```python
from build123d import *

# Parameters (mm, degrees)
F1_DEPTH        = 127
F3_DEPTH        = 25.4
F5_DEPTH        = 25.4
F12_DEPTH       = 3.1760001
F14_D           = 7.112
F14_CBORE_D     = 19.05
F14_CBORE_DEPTH = 6.35
F15_R           = 7.112
F15_R_2         = 4.445
F16_DEPTH       = 3.175
F17_R           = 7.112
F17_R_2         = 4.445
F18_DEPTH       = 3.175


with BuildPart() as f1:
    # F0 (on Top) → F1 (new body)
    with BuildSketch(Plane.XY):
        Polygon((-10.5701125115, 27.1786895925), (-17.3647849097, 0), (-14.0920698193, 0), (-8.0911474212, 24.0036895925), (8.0911474212, 24.0036895925), (14.0920698193, 0), (17.3647849097, 0), (10.5701125115, 27.1786895925), align=None)
    extrude(amount=F1_DEPTH)

    # F2 (on face) → F3 (join)
    with BuildSketch(Plane(origin=(0, 0, 0), x_dir=(1, 0, 0), z_dir=(0, 0, -1))):
        Polygon((8.0911474212, -24.0036895925), (14.0920698193, 0), (-14.0920698193, 0), (-8.0911474212, -24.0036895925), align=None)
        Polygon((17.3647849097, 0), (14.0920698193, 0), (8.0911474212, -24.0036895925), (-8.0911474212, -24.0036895925), (-14.0920698193, 0), (-17.3647849097, 0), (-10.5701125115, -27.1786895925), (10.5701125115, -27.1786895925), align=None)
    extrude(amount=F3_DEPTH)

    # F4 (on face) → F5 (join)
    with BuildSketch(Plane.XY.offset(127)):
        Polygon((-8.0911474212, 24.0036895925), (-14.0920698193, 0), (14.0920698193, 0), (8.0911474212, 24.0036895925), align=None)
        Polygon((-17.3647849097, 0), (-14.0920698193, 0), (-8.0911474212, 24.0036895925), (8.0911474212, 24.0036895925), (14.0920698193, 0), (17.3647849097, 0), (10.5701125115, 27.1786895925), (-10.5701125115, 27.1786895925), align=None)
    extrude(amount=F5_DEPTH)

    # F6 (on face) → F8 section 0
    with BuildSketch(Plane(origin=(16.3433269738, 4.0858317435, 0), x_dir=(-0.242535625, 0.9701425001, 0), z_dir=(0.9701425001, 0.242535625, 0))):
        Polygon((-4.2115789617, 158.75), (-4.2115789617, 152.4), (23.8035730273, 152.4), align=None)
    # F7 (on face) → F8 section 1
    with BuildSketch(Plane(origin=(-16.3433269738, 4.0858317435, 0), x_dir=(-0.242535625, -0.9701425001, 0), z_dir=(-0.9701425001, 0.242535625, 0))):
        Polygon((-23.8035730273, 152.4), (4.2115789617, 152.4), (4.2115789617, 158.75), align=None)
    loft()

    # F10 (on face) → F11 section 0
    with BuildSketch(Plane(origin=(-13.2631245358, 3.315781134, 0), x_dir=(0.242535625, 0.9701425001, 0), z_dir=(0.9701425001, -0.242535625, 0))):
        Polygon((-3.4178289617, 6.35), (-3.4178289617, 0), (21.324607937, 0), align=None)
    # F9 (on face) → F11 section 1
    with BuildSketch(Plane(origin=(13.2631245358, 3.315781134, 0), x_dir=(0.242535625, -0.9701425001, 0), z_dir=(-0.9701425001, -0.242535625, 0))):
        Polygon((-21.324607937, 0), (3.4178289617, 0), (3.4178289617, 6.35), align=None)
    loft()

    # F12 (cut, through all): a face of the model
    f12_faces = [f1.faces().sort_by_distance(p)[0] for p in [
        (0, 24.0036895925, 63.5),
    ]]
    extrude(f12_faces, amount=-F12_DEPTH, mode=Mode.SUBTRACT)

    # F14 (through all)
    with Locations(Plane(origin=(0, 27.1786895925, 0), x_dir=(-1, 0, 0), z_dir=(0, 1, 0))):
        with Locations((0, 139.7), (0, -12.7)):
            CounterBoreHole(F14_D / 2, F14_CBORE_D / 2, F14_CBORE_DEPTH)

    # F15 (on face) → F16 (join)
    with BuildSketch(Plane(origin=(16.3433269738, 4.0858317435, 0), x_dir=(-0.242535625, 0.9701425001, 0), z_dir=(0.9701425001, 0.242535625, 0))):
        with Locations((9.7959970328, 139.7)):
            Circle(F15_R)
        with Locations((9.7959970328, 139.7)):
            Circle(F15_R_2, mode=Mode.SUBTRACT)
        with Locations((9.7959970328, -12.7)):
            Circle(F15_R)
        with Locations((9.7959970328, -12.7)):
            Circle(F15_R_2, mode=Mode.SUBTRACT)
    extrude(amount=F16_DEPTH)

    # F17 (on face) → F18 (join)
    with BuildSketch(Plane(origin=(-16.3433269738, 4.0858317435, 0), x_dir=(-0.242535625, -0.9701425001, 0), z_dir=(-0.9701425001, 0.242535625, 0))):
        with Locations((-9.7959970328, 139.7)):
            Circle(F17_R)
        with Locations((-9.7959970328, 139.7)):
            Circle(F17_R_2, mode=Mode.SUBTRACT)
        with Locations((-9.7959970328, -12.7)):
            Circle(F17_R)
        with Locations((-9.7959970328, -12.7)):
            Circle(F17_R_2, mode=Mode.SUBTRACT)
    extrude(amount=F18_DEPTH)


solid = f1.part
```
Work out the finished part from the listing and answer in its coordinate system (mm). A direction names the side the tool comes from. Round coordinates to 2 decimals unless told otherwise and drop trailing zeros. Order: outer loops, then holes, each group sorted by start corner. A loop starts at its lowest first (then second) coordinate and runs counter-clockwise, first axis right, second up.
Q1. A cutting plane is placed at B-B, the plane x = 0. Count the separate pieces of the cut face and the enclosed holes in it, then the cut area to 3 significant figures.
Solution:
separate pieces: 4
enclosed holes: 0
area: 1,000 mm2
Q2. The mould has two halves that part along Y. Classify faces 4 (the flat face through (-9, 27.179, 63)), 5 (the flat face through (-15, 0, 88)), 6 (the cylindrical face through (-0.77, 10.27, 136.23)), 7 (the cylindrical face through (15.626, 13.408, -8.293)): pulls with the +Y half, pulls with the -Y half, needs draft (parallel to the pull), parting line crosses it, or undercut.
Solution:
face 4: pulls with the +Y half
face 5: pulls with the -Y half
face 6: needs draft
face 7: undercut
Q3. A tool of negligible diameter and unlimited length cuts with its end or side. For faces 1 (the flat face through (17.072, 14.263, -17.342)), 2 (the flat face through (-13.952, 13.65, 139.638)), 3 (the flat face through (-4, 20.829, 140)), from which of +Z, -Z, +X, -X, +Y, -Y can it reach the whole face along a straight path? Write none if from no direction.
Solution:
face 1: +Z, -Z, +X, +Y
face 2: none
face 3: +Y
Q4. A cutting plane is placed at D-D, the plane z = 139.7. Determine the outline of the cut face in (x, y) (3 decimals), then the cut area to 3 significant figures.
Solution:
outline: (-18.773, 7.46) - (-15.692, 6.69) - (-17.365, 0) - (-3.556, 0) - (-3.556, 20.829) - (-9.525, 20.829) - (-9.525, 27.179) - (-10.57, 27.179) - (-12.243, 20.489) - (-15.323, 21.259) - (-15.97, 18.672) - (-12.889, 17.902) - (-15.046, 9.277) - (-18.126, 10.047) - close; (3.556, 0) - (17.365, 0) - (15.692, 6.69) - (18.773, 7.46) - (18.126, 10.047) - (15.046, 9.277) - (12.889, 17.902) - (15.97, 18.672) - (15.323, 21.259) - (12.243, 20.489) - (10.57, 27.179) - (9.525, 27.179) - (9.525, 20.829) - (3.556, 20.829) - close
area: 524 mm2
Q5. Find the intervals of material crossed by line 1 along Z through (x, y) = (0, 6.25); line 2 along Z through (x, y) = (0, 25.5) (3 decimals); line 3 along X through (y, z) = (18.25, 73), in increasing order.
Solution:
line 1: z = -25.4 to -16.26, -9.14 to 4.7, 127 to 136.14, 143.26 to 157.29
line 2: z = -25.4 to -22.225, -3.175 to 0, 127 to 130.175, 149.225 to 152.792
line 3: x = -12.8 to -9.53, 9.53 to 12.8
Q6. A cutting plane is placed at A-A, the plane z = 51. Determine the outline of the cut face in (x, y), then the cut area to 3 significant figures.
Solution:
outline: (-17.36, 0) - (-14.09, 0) - (-8.09, 24) - (-8.09, 27.18) - (-10.57, 27.18) - close; (8.09, 24) - (14.09, 0) - (17.36, 0) - (10.57, 27.18) - (8.09, 27.18) - close
area: 175 mm2
Q7. Given pin 1 Ø1 at (y, z) = (25, 70.5) entering from +X; pin 2 Ø3 at (x, z) = (-5, 115.5) entering from -Y; pin 3 Ø9 at (x, z) = (0, 139.7) entering from +Y; pin 4 Ø2.5 at (y, z) = (25.5, 40.5) entering from -X, each flat-ended and moving along its own axis, determine where each tip first touches the part or whether it passes through.
Solution:
pin 1: stops at x = 11.24
pin 2: passes through
pin 3: stops at y = 20.83
pin 4: stops at x = -11.3
